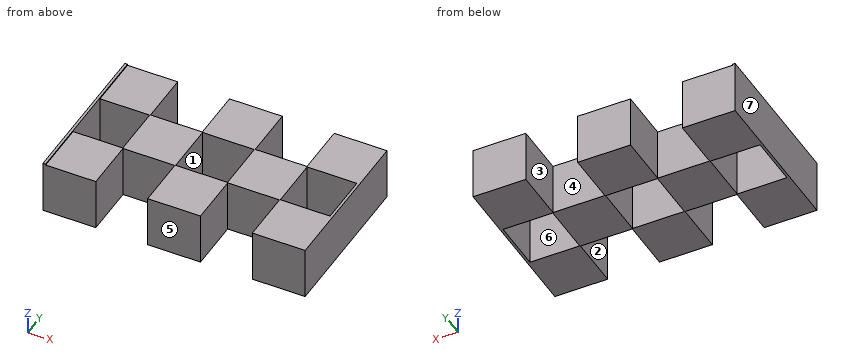
from build123d import *

# Parameters (mm, degrees)
F0_W      = 10.1
F0_H      = 10.1
F1_DEPTH  = 10.1
F9_W      = 30.1
F9_H      = 10.3136999533
F10_DEPTH = 0.5
F11_W     = 30.1
F11_H     = 10.1
F12_DEPTH = 0.5


with BuildPart() as f1:
    # F0 (on Top) → F1 (new body)
    with BuildSketch(Plane.XY):
        with Locations((5.05, 5.05)):
            Rectangle(F0_W, F0_H)
    extrude(amount=F1_DEPTH)


with BuildPart() as f2_1:
    # F2: copy of F1
    add(f1.part.moved(Location((20, 0, 0))))


with BuildPart() as f3_1:
    # F3: copy of F2_1
    add(f2_1.part.moved(Location((20, 0, 0))))


with BuildPart() as f4_1:
    # F4: copy of F1
    add(f1.part.moved(Location((10, 10, 0))))


with BuildPart() as f5_1:
    # F5: copy of F2_1
    add(f2_1.part.moved(Location((10, 10, 0))))


with BuildPart() as f6_1:
    # F6: copy of F4_1
    add(f4_1.part.moved(Location((-10, 10, 0))))


with BuildPart() as f7_1:
    # F7: copy of F4_1
    add(f4_1.part.moved(Location((10, 10, 0))))


with BuildPart() as f8_1:
    # F8: copy of F5_1
    add(f5_1.part.moved(Location((10, 10, 0))))


with BuildPart() as f1_1:
    add(f1.part)

    add(f6_1.part)  # F10 merges F6_1
    # F9 (on face) → F10 (join)
    with BuildSketch(Plane(origin=(0, 0, 0), x_dir=(0, -1, 0), z_dir=(-1, 0, 0))):
        with Locations((-15.05, 5.1568499766)):
            Rectangle(F9_W, F9_H)
    extrude(amount=-F10_DEPTH)

    add(f2_1.part)  # F12 merges F2_1

    add(f3_1.part)  # F12 merges F3_1

    add(f4_1.part)  # F12 merges F4_1

    add(f5_1.part)  # F12 merges F5_1

    add(f7_1.part)  # F12 merges F7_1

    add(f8_1.part)  # F12 merges F8_1
    # F11 (on face) → F12 (join)
    with BuildSketch(Plane.YZ.offset(50.1)):
        with Locations((15.05, 5.05)):
            Rectangle(F11_W, F11_H)
    extrude(amount=-F12_DEPTH)


solid = f1_1.part
Can you work these out from the model? Positions are in its coordinate system, mm. Face numbers are marked on the shaded views. A direction names the side the tool comes from. Give positions to 0.01 mm unless a question says otherwise; leave off trailing zeros. Order: outer loops, then holes, each group sorted by start corner. A loop starts at its lowest first (then second) coordinate and runs counter-clockwise, first axis right, second up. Notation, with made-up numbers: M -7.5,30 L 48.5,30 A36 cw 48.5,65 Z; hole C -23.5,-9.75 d1. An arc over 180 degrees is marked long. One line per item, written item: value.
Item 1: For pin 1 (4 mm diameter, centred on x = 34, y = 9, fed in from +Z); pin 2 (5 mm diameter, centred on x = 34.5, z = 5, fed in from -Y), each with a flat end and sliding along its axis, tell me the tip position at first contact or that it passes through.
Verdict:
pin 1: z = 10.1
pin 2: y = 10
Item 2: If we section it at D-D on y = 22: Write out the boundary of the cut face in (x, z), and give its area (3 significant figures).
Verdict:
outline: M 0,0 L 10.1,0 L 10.1,10.1 L 0.5,10.1 L 0.5,10.31 L 0,10.31 Z; M 20,0 L 30.1,0 L 30.1,10.1 L 20,10.1 Z; M 40,0 L 50.1,0 L 50.1,10.1 L 40,10.1 Z
area: 306 mm2
Item 3: If we mould it in two halves opening along Y, with no side actions, what happens to the marked faces 4, 5, 6 and 7? For each: pulls with the +Y half, pulls with the -Y half, needs draft (parallel to the pull), parting line crosses it, or undercut.
Verdict:
face 4: pulls with the +Y half
face 5: pulls with the -Y half
face 6: undercut
face 7: needs draft
Item 4: If we section it at A-A on x = 9.5: Write out the boundary of the cut face in (y, z).
Verdict:
outline: M 0,0 L 10.1,0 L 10.1,10.1 L 0,10.1 Z; M 20,0 L 30.1,0 L 30.1,10.1 L 20,10.1 Z
Item 5: If we section it at B-B on y = 12: Write out the boundary of the cut face in (x, z).
Verdict:
outline: M 0,0 L 0.5,0 L 0.5,10.31 L 0,10.31 Z; M 10,0 L 20.1,0 L 20.1,10.1 L 10,10.1 Z; M 30,0 L 40.1,0 L 40.1,10.1 L 30,10.1 Z; M 49.6,0 L 50.1,0 L 50.1,10.1 L 49.6,10.1 Z
Item 6: If we section it at C-C on z = 9: State how many separate pieces and enclosed holes the cut face has, and give its area (3 significant figures).
Verdict:
separate pieces: 1
enclosed holes: 3
area: 826 mm2
Item 7: Please list where these lines run through material, in increasing order: line 1 (X direction, y = 27, z = 3); line 2 (X direction, y = 13, z = 1.25); line 3 (Y direction, x = 46.5, z = 1.5).
Verdict:
line 1: 0 to 10.1, 20 to 30.1, 40 to 50.1
line 2: 0 to 0.5, 10 to 20.1, 30 to 40.1, 49.6 to 50.1
line 3: 0 to 10.1, 20 to 30.1
Item 8: For the marked faces 1, 2 and 3, which set-ups out of +Z, -Z, +X, -X, +Y, -Y let a thin tool reach every point of the face, with its end or its side?
Verdict:
face 1: +Z, -Z
face 2: +Z, -Z, -Y
face 3: +Z, -Z, +Y
